Autodesk Inventor part; units mm, degrees
ref_plane "YZ Plane" through (0, 0, 0) normal (1, 0, 0) x (0, 1, 0)
ref_plane "XZ Plane" through (0, 0, 0) normal (0, 1, 0) x (-1, 0, 0)
ref_plane "XY Plane" through (0, 0, 0) normal (0, 0, 1) x (1, 0, 0)
sketch "Sketch1" plane through (0, 0, 0) normal (1, 0, 0) x (0, 1, 0)
  circle A0 centre (-0.038, 0) radius 1.5
  point P0 (0, 0)
  dimension "d0" = 3
extrude "Extrusion1" add sketch "Sketch1" along normal blind 15
sketch "Sketch2" plane through (15, -0.038, 0) normal (1, 0, 0) x (0, 0, -1)
  circle A0 centre (0, 0) radius 1.5
  line L0 (-0.1729, 1.49) -> (0.1729, 1.49)
  point P0 (0, 0.038)
  point P1 (0, 1.49)
  dimension "d3" = 1.49
extrude "Extrusion2" cut sketch "Sketch2" against normal blind 1 contours L0 A0 picked at (-0.0192, 1.493)
sketch "Sketch3" plane through (15, 0, 0) normal (1, 0, 0) x (0, 0, -1)
  point P0 (0, 0)
sketch "Sketch4" plane through (15, 0, 0) normal (1, 0, 0) x (0, 0, -1)
  arc A0 (-0.1729, 1.452) -> (0.1729, 1.452) centre (0, -0.038) ccw
  line L0 (-1.49, 0.135) -> (-1.49, -0.2109)
  line L1 (0.1729, 1.452) -> (-0.1729, 1.452)
  point P0 (0, 0)
  point P1 (-1.49, -0.038)
  dimension "d6" = 1.49
extrude "Extrusion3" cut sketch "Sketch4" against normal blind 1 contours L0 A0
properties part number "pin" material "Steel"
CAD build for the part. Positions are in the model's coordinates, mm. Round coordinates to 2 decimals unless told otherwise and drop trailing zeros. Write each loop counter-clockwise with the first axis right and the second up, starting at its lowest first coordinate (ties: lowest second). Pieces come first, ordered by that corner, then holes. Notation, with made-up numbers: (88.25, 48.5) - (104.25, 48.5) arc R8 cw to (104.25, 61.5) - close; hole circle Ø9 at (21.5, 89). An arc over 180 degrees is marked (long way). Write item = value, one per line. Start each with the question number.
Q1. Probe L1, parallel to Z at x = 13, y = -1.3; L2, parallel to Z at x = 10.75, y = -0.9; L3, parallel to Y at x = 13.5, z = -0.85. List the from-to ranges inside material, lowest first. Write a range as from..to.
Q2. Band-saw the part on C-C (z = 0.85). Give the cut face in (x, y), then the cut area to 3 significant figures.
Q3. Band-saw the part on A-A (x = 5). Give the cut face in (y, z).
Q4. Band-saw the part on B-B (y = 1.15). Give the cut face in (x, z), then the cut area to 3 significant figures.
Answers below:
q1.L1 = -0.81..0.81
q1.L2 = -1.23..1.23
q1.L3 = -1.27..1.2
q2.outline = (0, -1.27) - (15, -1.27) - (15, 1.2) - (0, 1.2) - close
q2.area = 37.1 mm2
q3.outline = circle Ø3 at (-0.04, 0)
q4.outline = (0, -0.92) - (15, -0.92) - (15, 0.92) - (0, 0.92) - close
q4.area = 27.5 mm2
